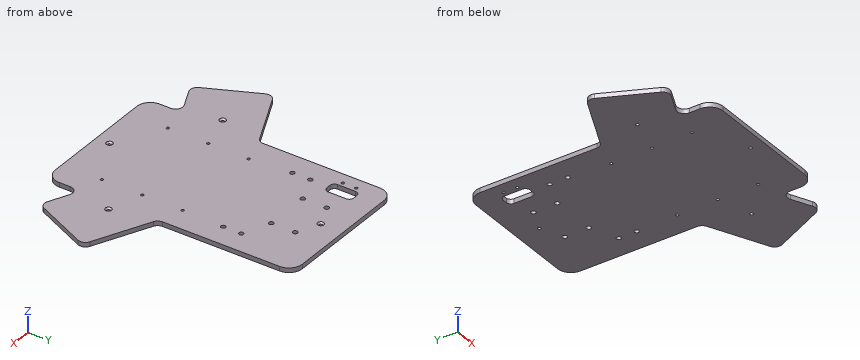
Solid Edge part; units mm, degrees
sketch "Sketch1" plane through (0, 0, 0) normal (0, 0, 1) x (1, 0, 0)
  line L0 (-30, 165) -> (-30, -80)
  arc A0 (-15, -95) -> (-30, -80) centre (-15, -80) cw
  line L1 (-15, -95) -> (115, -95)
  arc A1 (130, -80) -> (115, -95) centre (115, -80) cw
  line L2 (130, -80) -> (130, 165)
  arc A2 (115, 180) -> (130, 165) centre (115, 165) cw
  line L3 (115, 180) -> (-15, 180)
  arc A3 (-15, 180) -> (-30, 165) centre (-15, 165) ccw
extrude "Protrusion1" add sketch "Sketch1" against normal blind 5
sketch "Sketch2" plane through (0, 0, 0) normal (0, 0, 1) x (1, 0, 0)
  circle A0 centre (50, 155) radius 1.8
extrude "Cutout1" cut sketch "Sketch2" against normal through all
sketch "Sketch3" plane through (65, 80, 0) normal (0, 0, 1) x (1, 0, 0)
  circle A0 centre (-70, 25) radius 2.5
  circle A1 centre (-70, 5) radius 2.5
  circle A2 centre (40, 25) radius 2.5
  circle A3 centre (40, 5) radius 2.5
  line L0 (-62.5, 50) -> (-62.5, 70)
  arc A4 (-67.5, 75) -> (-62.5, 70) centre (-67.5, 70) cw
  line L1 (-67.5, 75) -> (-72.5, 75)
  arc A5 (-72.5, 75) -> (-77.5, 70) centre (-72.5, 70) ccw
  line L2 (-77.5, 70) -> (-77.5, 50)
  arc A6 (-77.5, 50) -> (-72.5, 45) centre (-72.5, 50) ccw
  line L3 (-72.5, 45) -> (-67.5, 45)
  arc A7 (-62.5, 50) -> (-67.5, 45) centre (-67.5, 50) cw
extrude "Cutout2" cut sketch "Sketch3" against normal through all
sketch "Sketch4" plane through (50, 42.5, 0) normal (0, 0, 1) x (1, 0, 0)
  line L0 (80, -12.4898) -> (152.5689, -46.1611)
  line L1 (152.5689, -46.1611) -> (119.855, -116.316)
  line L2 (80, -97.9097) -> (119.855, -116.316)
  line L3 (80, -12.4898) -> (80, -97.9097)
  line L4 (-152.57, -46.1587) -> (-80, -12.4898)
  line L5 (-80, -12.4898) -> (-80, -97.9098)
  line L6 (-80, -97.9098) -> (-119.855, -116.316)
  line L7 (-119.855, -116.316) -> (-152.57, -46.1587)
extrude "Protrusion2" add sketch "Sketch4" against normal blind 5
fillet "Round_1" radius 8 8 edges at (202.5689, -3.6611, -2.5) (169.855, -73.816, -2.5) (130, -55.4097, -2.5) (130, 30.0102, -2.5) (-30, 30.0102, -2.5) (-102.57, -3.6587, -2.5) (-69.855, -73.816, -2.5) (-30, -55.4098, -2.5)
sketch "Sketch5" plane through (49.9995, 42.5, 0) normal (0, 0, 1) x (1, 0, 0)
  circle A0 centre (-90.8872, -60.1268) radius 1.8
  circle A1 centre (0.0005, -122.5) radius 1.8
  circle A2 centre (90.8881, -60.1268) radius 1.8
extrude "Cutout3" cut sketch "Sketch5" against normal up to next
chamfer "Chamfer_3" distance 1.67 angle 45 4 edges at (-42.6876, -17.6268, 0) (48.2, -80, 0) (139.0876, -17.6268, 0) (48.2, 155, 0)
sketch "Sketch6" plane through (49.9995, 42.5, 0) normal (0, 0, 1) x (1, 0, 0)
  circle A0 centre (-67.3495, 105) radius 1.6
  circle A1 centre (-67.3495, 90) radius 1.6
extrude "Cutout4" cut sketch "Sketch6" against normal up to next
sketch "Sketch7" plane through (49.9995, 42.5, 0) normal (0, 0, 1) x (1, 0, 0)
  circle A0 centre (-24.9995, 101.5) radius 2.65
  circle A1 centre (25.0005, 101.5) radius 2.65
  circle A2 centre (-24.9995, 74.97) radius 2.65
  circle A3 centre (25.0005, 74.97) radius 2.65
extrude "Cutout5" cut sketch "Sketch7" against normal up to next
sketch "Sketch8" plane through (49.9995, 42.5, 0) normal (0, 0, 1) x (1, 0, 0)
  circle A0 centre (-51.2495, -93.5) radius 1.5
  circle A1 centre (-51.2495, -48.5) radius 1.5
  circle A2 centre (-51.2495, -3.5) radius 1.5
  circle A3 centre (53.7505, -3.5) radius 1.5
  circle A4 centre (53.7505, -48.5) radius 1.5
  circle A5 centre (53.7505, -93.5) radius 1.5
extrude "Cutout6" cut sketch "Sketch8" against normal up to next
properties material "Polycarbonate( 20-40% Glass Fiber)"
Source: CAD feature listing. Evaluate the final solid. Frame: model axes, mm. Give positions to 0.01 mm unless a question says otherwise; leave off trailing zeros. Loops run counter-clockwise (first coordinate to the right, second up) from the corner with the lowest first, then second, coordinate; pieces in that order, holes last. Notation, with made-up numbers: (72, -33) - (126, -33) arc R16 ccw to (126, -26) - close; hole circle Ø2 at (7.25, 13). An arc over 180 degrees is marked (long way). Use CSV: the item, a comma, the result in double quotes.
1) Cut plane A-A (z = -2.5). Count the separate pieces of the cut face and the enclosed holes in it, and give its area (3 significant figures).
Worked out:
separate pieces,"1"
enclosed holes,"21"
area,"52,700 mm^2"
2) Line query: line 1 (Y direction, x = 25, z = -2.5); line 2 (X direction, y = 147.5, z = -3.4); line 3 (X direction, y = 144, z = -1.6). Output: solid intervals per line, ascending.
Worked out:
line 1,"y = -95 to 114.82, 120.12 to 141.35, 146.65 to 180"
line 2,"x = -30 to -18.95, -15.75 to -12.5, 2.5 to 130"
line 3,"x = -30 to -12.5, 2.5 to 22.35, 27.65 to 72.35, 77.65 to 130"
3) Cut plane B-B (y = -33.5). Output: boundary loops of the cut face in (x, z).
Worked out:
outline,"(-88.65, -5) - (188.65, -5) - (188.65, 0) - (-88.65, 0) - close"
4) Pin query (flat end, axial travel): P1, Ø1.9, axis at x = -17.35, y = 132.5, coming from the -Z side; P2, Ø2.5, axis at y = 140.5, z = -1.5, coming from the +X side; P3, Ø2, axis at x = 139, z = -3, coming from the +Y side; P4, Ø2, axis at y = -15.5, z = -1, coming from the -X side. Return the tip coordinate at first contact, or that it passes through.
Worked out:
P1,"passes through"
P2,"stops at x = 130"
P3,"stops at y = 26.3"
P4,"stops at x = -97.51"
5) Cut plane C-C (y = 20.5). Output: boundary loops of the cut face in (x, z), and give its area (3 significant figures).
Worked out:
outline,"(-50.5, -5) - (150.5, -5) - (150.5, 0) - (-50.5, 0) - close"
area,"1,000 mm^2"
